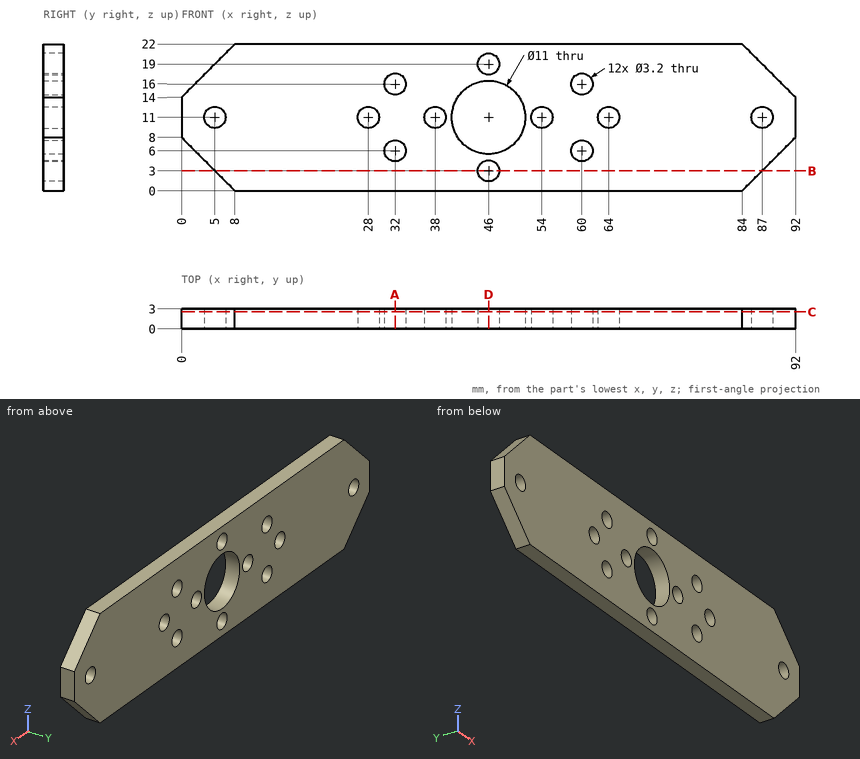
The drawing under review shows one solid part. Ordinate dimensions are in mm from its lowest x, y, z. Round coordinates to 2 decimals unless told otherwise and drop trailing zeros. Write each loop counter-clockwise with the first axis right and the second up, starting at its lowest first coordinate (ties: lowest second). Pieces come first, ordered by that corner, then holes. Notation, with made-up numbers: (72, -37) -> (92, -37) arc R11 cw to (92, -16) -> close; hole circle Ø11 at (19.5, 25). An arc over 180 degrees is marked (long way). One line per question, with ' | ' between items.
(1) Take a section at B-B, the plane z = 3. State the section outline as (x, y) points.
Result sheet:
outline: (5, 0) -> (44.4, 0) -> (44.4, 3) -> (5, 3) -> close; (47.6, 0) -> (87, 0) -> (87, 3) -> (47.6, 3) -> close
(2) Insertion check: P1, Ø1.5, axis at y = 2, z = 15, coming from the +X side. The pin has a flat end and moves straight along its axis. Give the tip position at first contact, or say it passes through.
Result sheet:
P1: x = 91.75
(3) Take a section at C-C, the plane y = 2.55. State how many separate pieces and enclosed holes the cut face has, and give its area (3 significant figures).
Result sheet:
separate pieces: 1 | enclosed holes: 13 | area: 1,700 mm2
(4) Take a section at A-A, the plane x = 32. State the section outline as (y, z) points.
Result sheet:
outline: (0, 0) -> (3, 0) -> (3, 4.4) -> (0, 4.4) -> close; (0, 7.6) -> (3, 7.6) -> (3, 14.4) -> (0, 14.4) -> close; (0, 17.6) -> (3, 17.6) -> (3, 22) -> (0, 22) -> close
(5) Take a section at D-D, the plane x = 46. State the section outline as (y, z) points, and give its area (3 significant figures).
Result sheet:
outline: (0, 0) -> (3, 0) -> (3, 1.4) -> (0, 1.4) -> close; (0, 4.6) -> (3, 4.6) -> (3, 5.5) -> (0, 5.5) -> close; (0, 16.5) -> (3, 16.5) -> (3, 17.4) -> (0, 17.4) -> close; (0, 20.6) -> (3, 20.6) -> (3, 22) -> (0, 22) -> close | area: 13.8 mm2
(6) Wall thickness on line 1 (X direction, y = 2.45, z = 17); line 2 (X direction, y = 1.1, z = 6); line 3 (Z direction, x = 31, y = 0.55): over which ranges is each line inside the solid? List them lowest first. Write a range as [from, to].
Result sheet:
line 1: [3, 30.75], [33.25, 58.75], [61.25, 89] | line 2: [2, 30.4], [33.6, 43.71], [48.29, 58.4], [61.6, 90] | line 3: [0, 4.75], [7.25, 14.75], [17.25, 22]
